Autodesk Inventor part; units mm, degrees
ref_plane "YZ Plane" through (0, 0, 0) normal (1, 0, 0) x (0, 1, 0)
ref_plane "XZ Plane" through (0, 0, 0) normal (0, 1, 0) x (-1, 0, 0)
ref_plane "XY Plane" through (0, 0, 0) normal (0, 0, 1) x (1, 0, 0)
sketch "Sketch1" plane through (0, 0, 0) normal (0, 0, 1) x (1, 0, 0)
  circle A0 centre (0, 0) radius 9.525
  dimension "d8" = 19.05
extrude "Extrusion1" add sketch "Sketch1" against normal blind 38.1
sketch "Sketch2" plane through (0, 0, 0) normal (0, 0, 1) x (1, 0, 0)
  circle A0 centre (0, 0) radius 2.3813
  dimension "d2" = 4.7625
extrude "Extrusion2" add sketch "Sketch2" along normal blind 25.4
sketch "Sketch4" plane through (0, 0, -38.1) normal (0, 0, -1) x (-1, 0, 0)
  circle A0 centre (0, 0) radius 4
  dimension "d5" = 8
extrude "Extrusion3" cut sketch "Sketch4" against normal blind 31.75
properties part number "CIM to 0_1875 Worm Gearn"
Read the model definition and answer for the solid it produces. Units are mm, in the model's axes. A direction names the side the tool comes from. Round coordinates to 2 decimals unless told otherwise and drop trailing zeros. Loops run counter-clockwise (first coordinate to the right, second up) from the corner with the lowest first, then second, coordinate; pieces in that order, holes last.
Q1. Which of the six approach directions +Z, -Z, +X, -X, +Y, -Y give full straight-line access (tool end or side, diameter ignored) to faces 4 (the face through (0.867, -3.905, -22.447)), 5 (the face through (0, 0, 25.4))?
Q2. Section A-A on x = 0 is taken. Write down the section's boundary in (y, z) (3 decimals).
Q3. Section B-B on z = -28 is taken. Write down the section's boundary in (x, y) (3 decimals), and give its area (3 significant figures).
Q4. Section D-D on z = -3 is taken. Write down the section's boundary in (x, y) (3 decimals), and give its area (3 significant figures).
Q5. Consider probe 1 along Z at (x, y) = (8.5, -2.75); probe 2 along Y at (x, z) = (0, -23.5) (3 decimals); probe 3 along Z at (x, y) = (3.5, -1). Determine where each line is inside the solid, lowest interval first.
Q6. Each of these flat-tipped pins is pushed along its axis until it touches: pin 1 (2 mm diameter, centred on x = -4, y = 5.5, fed in from +Z); pin 2 (2 mm diameter, centred on y = 1.5, z = -8.5, fed in from -X); pin 3 (6.5 mm diameter, centred on x = -1, y = 1.5, fed in from -Z); pin 4 (2 mm diameter, centred on y = -3.5, z = -19.5, fed in from +X). Where does it stop, or does it pass through?
Q7. Determine the mould class of faces 1 (the face through (2, -2, 0)), 2 (the face through (1.1, 2.11, 12.52)), 3 (the face through (0, 0, -6.35)) for opening direction X: released by +X, released by -X, zero draft, split by the parting line, or undercut.
Output:
1. face 4: -Z
1. face 5: +Z, +X, -X, +Y, -Y
2. outline: (-9.525, -38.1) - (-4, -38.1) - (-4, -6.35) - (4, -6.35) - (4, -38.1) - (9.525, -38.1) - (9.525, 0) - (2.381, 0) - (2.381, 25.4) - (-2.381, 25.4) - (-2.381, 0) - (-9.525, 0) - close
3. outline: circle Ø19.05 at (0, 0); hole circle Ø8 at (0, 0)
3. area: 235 mm2
4. outline: circle Ø19.05 at (0, 0)
4. area: 285 mm2
5. probe 1: z = -38.1 to 0
5. probe 2: y = -9.525 to -4, 4 to 9.525
5. probe 3: z = -6.35 to 0
6. pin 1: stops at z = 0
6. pin 2: stops at x = -9.51
6. pin 3: stops at z = -38.1
6. pin 4: stops at x = 9.19
7. face 1: zero draft
7. face 2: split by the parting line
7. face 3: undercut
